Build history of the part. All positions in model axes, mm. A direction names the side the tool comes from. Round coordinates to 2 decimals unless told otherwise and drop trailing zeros. Order: outer loops, then holes, each group sorted by start corner. A loop starts at its lowest first (then second) coordinate and runs counter-clockwise, first axis right, second up. Notation, with made-up numbers: M 66,88 L 95,88 A17 cw 95,104 Z; hole C -27,47.5 d3. An arc over 180 degrees is marked long. One line per item, written item: value. Start each with the question number.
Item 1: Probe L1, parallel to X at y = 100, z = -12; L2, parallel to X at y = 63, z = -3; L3, parallel to Z at x = -18.5, y = 66.5. List the from-to ranges inside material, lowest first.
Item 2: Band-saw the part on A-A, the plane y = 37. Write the cut outline in (x, z), then the cut area to 3 significant figures.
Item 3: Two-plate mould, pull along Z, no slides. Class faces 1 (the flat face through (-5.883, 56, -17)), 2 (the cylindrical face through (-18.443, 54.23, -38.287)), 3 (the flat face through (-38.883, 54, -8)): +Z half, -Z half, draft (parallel to the pull), parting line (faces both ways), or undercut.
Item 4: Band-saw the part on D-D, the plane x = -2. Write the cut outline in (y, z).
Item 5: Band-saw the part on B-B, the plane y = 55. Write the cut outline in (x, z).
Item 6: Band-saw the part on C-C, the plane z = -14. Write the cut outline in (x, y).
Item 7: Tool access for faces 4 (the cylindrical face through (-38.39, 52.193, -5.582)), 5 (the flat face through (-3, 56, -16.292)), 6 (the flat face through (1.117, 54, -8)): list every direction of +Z, -Z, +X, -X, +Y, -Y with a clear straight run to the whole face (end or side of a thin tool).
Item 8: Pin check, flat tips, straight feed: pin 1 (6.5 mm diameter, centred on x = -1.5, y = 62, fed in from -Z); pin 2 (12 mm diameter, centred on x = -28, z = -17, fed in from +Y); pin 3 (1.5 mm diameter, centred on y = 65, z = -32, fed in from +X); pin 4 (3 mm diameter, centred on x = -15.5, z = -15, fed in from +Y). Stop position of each tip, or through.
```python
from build123d import *

# Parameters (mm, degrees)
BOSS_EXTRUDE1_DEPTH = 110
CUT_EXTRUDE1_DEPTH  = 109
SKETCH3_R           = 2.875
CUT_EXTRUDE2_DEPTH  = 5


with BuildPart() as part:
    # Sketch1 → Boss-Extrude1 (new body)
    with BuildSketch(Plane(origin=(0, 0, 0), x_dir=(1, 0, 0), z_dir=(0, 1, 0))):
        with BuildLine():
            Line((-38.883093525, -1.707733813), (1.116906475, -1.707733813))
            Line((1.116906475, -1.707733813), (1.116906475, 18.292266187))
            ThreePointArc((1.116906475, 18.292266187), (-18.883093525, 38.292266187), (-38.883093525, 18.292266187))
            Line((-38.883093525, 18.292266187), (-38.883093525, -1.707733813))
        make_face()
    extrude(amount=BOSS_EXTRUDE1_DEPTH)

    # Sketch2 → Cut-Extrude1 (cut)
    with BuildSketch(Plane(origin=(0, 110, 0), x_dir=(1, 0, 0), z_dir=(0, 1, 0))):
        with BuildLine():
            Line((-37.883093525, 16.292266187), (-37.883093525, 12.292266187))
            Line((-37.883093525, 12.292266187), (-31.883093525, 12.292266187))
            Line((-31.883093525, 12.292266187), (-31.883093525, 10.292266187))
            Line((-31.883093525, 10.292266187), (-37.883093525, 10.292266187))
            Line((-37.883093525, 10.292266187), (-37.883093525, -0.707733813))
            Line((-37.883093525, -0.707733813), (0.116906475, -0.707733813))
            Line((0.116906475, -0.707733813), (0.116906475, 10.292266187))
            Line((0.116906475, 10.292266187), (-5.883093525, 10.292266187))
            Line((-5.883093525, 10.292266187), (-5.883093525, 12.292266187))
            Line((-5.883093525, 12.292266187), (0.116906475, 12.292266187))
            Line((0.116906475, 12.292266187), (0.116906475, 16.292266187))
            Line((0.116906475, 16.292266187), (-5.883093525, 16.292266187))
            Line((-5.883093525, 16.292266187), (-5.883093525, 18.292266187))
            Line((-5.883093525, 18.292266187), (0.116906475, 18.292266187))
            ThreePointArc((0.116906475, 18.292266187), (-18.883093525, 37.292266187), (-37.883093525, 18.292266187))
            Line((-37.883093525, 18.292266187), (-31.883093525, 18.292266187))
            Line((-31.883093525, 18.292266187), (-31.883093525, 16.292266187))
            Line((-31.883093525, 16.292266187), (-37.883093525, 16.292266187))
        make_face()
    extrude(amount=-CUT_EXTRUDE1_DEPTH, mode=Mode.SUBTRACT)

    # Sketch3 → Cut-Extrude2 (cut)
    with BuildSketch(Plane.ZY.offset(38.883093525)):
        with Locations((-4.958932854, 55)):
            Circle(SKETCH3_R)
    extrude(amount=-CUT_EXTRUDE2_DEPTH, mode=Mode.SUBTRACT)


solid = part.part
```
Output:
1. L1: x = -38.88 to -31.88, -5.88 to 1.12
1. L2: x = -38.88 to -37.88, 0.12 to 1.12
1. L3: z = -38.29 to -37.29, 0.71 to 1.71
2. outline: M -38.88,-18.29 A20 ccw 1.12,-18.29 L 1.12,1.71 L -38.88,1.71 Z; hole M -37.88,-18.29 A19 ccw 0.12,-18.29 L -5.88,-18.29 L -5.88,-16.29 L 0.12,-16.29 L 0.12,-12.29 L -5.88,-12.29 L -5.88,-10.29 L 0.12,-10.29 L 0.12,0.71 L -37.88,0.71 L -37.88,-10.29 L -31.88,-10.29 L -31.88,-12.29 L -37.88,-12.29 L -37.88,-16.29 L -31.88,-16.29 L -31.88,-18.29 Z
2. area: 187 mm²
3. face 1: undercut
3. face 2: -Z half
3. face 3: draft
4. outline: M 0,-29.01 L 110,-29.01 L 110,-27.01 L 1,-27.01 L 1,-18.29 L 110,-18.29 L 110,-16.29 L 1,-16.29 L 1,-12.29 L 110,-12.29 L 110,-10.29 L 1,-10.29 L 1,0.71 L 110,0.71 L 110,1.71 L 0,1.71 Z
5. outline: M -38.88,-18.29 A20 ccw 1.12,-18.29 L 1.12,1.71 L -38.88,1.71 L -38.88,-2.08 L -37.88,-2.08 L -37.88,0.71 L 0.12,0.71 L 0.12,-10.29 L -5.88,-10.29 L -5.88,-12.29 L 0.12,-12.29 L 0.12,-16.29 L -5.88,-16.29 L -5.88,-18.29 L 0.12,-18.29 A19 cw -37.88,-18.29 L -31.88,-18.29 L -31.88,-16.29 L -37.88,-16.29 L -37.88,-12.29 L -31.88,-12.29 L -31.88,-10.29 L -37.88,-10.29 L -37.88,-7.83 L -38.88,-7.83 Z
6. outline: M -38.88,0 L 1.12,0 L 1.12,110 L 0.12,110 L 0.12,1 L -37.88,1 L -37.88,110 L -38.88,110 Z
7. face 4: -X
7. face 5: +Y
7. face 6: +Z, -Z, +X, +Y, -Y
8. pin 1: stops at z = -32.44
8. pin 2: stops at y = 110
8. pin 3: stops at x = -3.65
8. pin 4: stops at y = 1
